```python
from build123d import *

# Parameters (mm, degrees)
SKETCH_1_R                   = 13.5
EXTRUDE_1_DEPTH              = 6
EXTRUDE_START                = -3.8
SKETCH_2_R                   = 19
SKETCH_2_R_2                 = 13.5
EXTRUDE_2_DEPTH              = 3.8
HOLE_WIZARD_M3_1_D           = 3.2
HOLE_WIZARD_M3_1_DEPTH       = 7
HOLE_WIZARD_M3_1_CSINK_D     = 6.5
HOLE_WIZARD_M3_1_CSINK_ANGLE = 90
HOLE_WIZARD_M3_1_TIP         = 0.96137699
F_2_0MM_1_D                  = 2
F_2_0MM_1_DEPTH              = 3.3
F_2_0MM_1_TIP                = 0.600860619
HOLE_WIZARD_M3_1_2_OUTLINE_R = 1.25
HOLE_WIZARD_M3_1_2_DEPTH     = 6
CUT_EXTRUDE_1_DEPTH          = 2
SKETCH_12_R                  = 17.5
SKETCH_12_R_2                = 14.5
CUT_EXTRUDE_3_DEPTH          = 2
EXTRUDE_START_2              = 2
EXTRUDE_3_DEPTH              = 2
CHAMFER_1_SIZE               = 0.5
FILLET_2_R                   = 1
CHAMFER_2_SIZE               = 0.5
CHAMFER_2_SIZE2              = 0.866025404
CHAMFER_3_SIZE               = 0.5


# Read off the part's stored shape, not the designer's step: M3 螺纹孔1
with BuildPart() as part:
    # 草图1 → 凸台-拉伸1 (new body)
    with BuildSketch(Plane.XY):
        Circle(SKETCH_1_R)
    extrude(amount=EXTRUDE_1_DEPTH)

    # 草图2 → 凸台-拉伸2 (add)
    with BuildSketch(Plane.XY.offset(6).offset(EXTRUDE_START)):
        Circle(SKETCH_2_R)
        Circle(SKETCH_2_R_2, mode=Mode.SUBTRACT)
    extrude(amount=EXTRUDE_2_DEPTH)

    # Hole Wizard M3 _1
    with Locations(Plane.XY.offset(6)):
        with Locations((8.660254038, -5), (0, 10), (-8.660254038, -5)):
            CounterSinkHole(HOLE_WIZARD_M3_1_D / 2, HOLE_WIZARD_M3_1_CSINK_D / 2, depth=HOLE_WIZARD_M3_1_DEPTH, counter_sink_angle=HOLE_WIZARD_M3_1_CSINK_ANGLE)
            with Locations((0, 0, -(HOLE_WIZARD_M3_1_DEPTH + HOLE_WIZARD_M3_1_TIP / 2))):  # 118° drill point
                Cone(0, HOLE_WIZARD_M3_1_D / 2, HOLE_WIZARD_M3_1_TIP, mode=Mode.SUBTRACT)

    # Ø2.0mm 暗销孔1
    with Locations(Plane(origin=(0, 0, 0), x_dir=(-1, 0, 0), z_dir=(0, 0, -1))):
        with Locations((8.660254038, 5), (0, -10), (-8.660254038, 5)):
            Hole(F_2_0MM_1_D / 2, depth=F_2_0MM_1_DEPTH)
            with Locations((0, 0, -(F_2_0MM_1_DEPTH + F_2_0MM_1_TIP / 2))):  # 118° drill point
                Cone(0, F_2_0MM_1_D / 2, F_2_0MM_1_TIP, mode=Mode.SUBTRACT)

    # Hole Wizard M3 _1 2 outline → Hole Wizard M3 _1 2 (cut)
    with BuildSketch(Plane.XY):
        with Locations((5.25, 0)):
            Circle(HOLE_WIZARD_M3_1_2_OUTLINE_R)
        with Locations((0, -5.25)):
            Circle(HOLE_WIZARD_M3_1_2_OUTLINE_R)
        with Locations((-5.25, 0)):
            Circle(HOLE_WIZARD_M3_1_2_OUTLINE_R)
        with Locations((0, 5.25)):
            Circle(HOLE_WIZARD_M3_1_2_OUTLINE_R)
    extrude(amount=HOLE_WIZARD_M3_1_2_DEPTH, mode=Mode.SUBTRACT)

    # 草图10 → 切除-拉伸1 (cut)
    with BuildSketch(Plane.XY.offset(6)):
        with BuildLine():
            Line((-2, -1), (-2, 1))
            ThreePointArc((-2, 1), (0, 3), (2, 1))
            Line((2, 1), (2, -1))
            ThreePointArc((2, -1), (0, -3), (-2, -1))
        make_face()
    extrude(amount=-CUT_EXTRUDE_1_DEPTH, mode=Mode.SUBTRACT)

    # 草图12 → 切除-拉伸3 (cut)
    with BuildSketch(Plane(origin=(0, 0, 2.2), x_dir=(-1, 0, 0), z_dir=(0, 0, -1))):
        Circle(SKETCH_12_R)
        Circle(SKETCH_12_R_2, mode=Mode.SUBTRACT)
    extrude(amount=-CUT_EXTRUDE_3_DEPTH, mode=Mode.SUBTRACT)

    # 草图13 → 凸台-拉伸3 (add)
    with BuildSketch(Plane(origin=(0, 0, 4.2), x_dir=(-1, 0, 0), z_dir=(0, 0, -1)).offset(EXTRUDE_START_2)):
        with BuildLine():
            Line((-2.517898576, 14.279712419), (-3.038843109, 17.234135678))
            ThreePointArc((-3.038843109, 17.234135678), (0, 17.5), (3.038843109, 17.234135678))
            Line((3.038843109, 17.234135678), (2.517898576, 14.279712419))
            ThreePointArc((2.517898576, 14.279712419), (0, 14.5), (-2.517898576, 14.279712419))
        make_face()
    extrude(amount=-EXTRUDE_3_DEPTH)

    # 倒角1
    chamfer_1_edges = [part.edges().sort_by_distance(p)[0] for p in [
        (-9.660254038, 5, 0),
        (-1, -10, 0),
        (7.660254038, 5, 0),
    ]]
    chamfer(chamfer_1_edges, length=CHAMFER_1_SIZE)

    # 圆角2
    fillet_2_edges = [part.edges().sort_by_distance(p)[0] for p in [
        (3.038843109, 17.234135678, 3.2),
        (-3.038843109, 17.234135678, 3.2),
        (-2.517898576, 14.279712419, 3.2),
        (2.517898576, 14.279712419, 3.2),
    ]]
    fillet(fillet_2_edges, radius=FILLET_2_R)

    # 倒角2
    chamfer_2_edges = [part.edges().sort_by_distance(p)[0] for p in [
        (0, -3, 6),
        (2, 0, 6),
        (0, 3, 6),
        (-2, 0, 6),
    ]]
    chamfer_2_side = [part.faces().sort_by_distance(p)[0] for p in [
        (-18.462598846, 0, 6),
    ]]
    chamfer(chamfer_2_edges, length=CHAMFER_2_SIZE, length2=CHAMFER_2_SIZE2, reference=chamfer_2_side[0])

    # 倒角3
    chamfer_3_edges = [part.edges().sort_by_distance(p)[0] for p in [
        (-2.772933692, 15.726088432, 2.2),
        (0, -14.5, 2.2),
        (0, -17.5, 2.2),
        (2.772933692, 15.726088432, 2.2),
        (-2.833509711, 14.512231288, 2.2),
        (-3.296257199, 16.88197424, 2.2),
        (3.296257199, 16.88197424, 2.2),
        (2.833509711, 14.512231288, 2.2),
        (-13.5, 0, 0),
        (-19, 0, 2.2),
        (-19, 0, 6),
    ]]
    chamfer(chamfer_3_edges, length=CHAMFER_3_SIZE)


solid = part.part
```
For this review, take the finished solid that the model builds, in its own axes (mm). A direction names the side the tool comes from. Give positions to 0.01 mm unless a question says otherwise; leave off trailing zeros. Answer as a JSON object with one key per item and string values. Group by question number.
Item 1: Consider section A-A on z = 1.45. Count the separate pieces of the cut face and the enclosed holes in it, plus the area to 3 significant figures.
Item 2: For probe 1 along Y at (x, z) = (0, 3.25); probe 2 along Y at (x, z) = (0, 1.2); probe 3 along X at (y, z) = (5, 2.7), list the stretches that pass through material, from the lowest coordinate up. Write a range as [from, to].
Item 3: For pin 1 Ø1.8 at (x, y) = (-8.66, 5) entering from -Z; pin 2 Ø2.5 at (x, y) = (8.66, 5) entering from -Z; pin 3 Ø1 at (y, z) = (12, 4) entering from +X, all flat-tipped, find the tip position at first contact; note any pin that passes through.
Item 4: Tool access review of faces 1 (the flat face through (-2.774, 15.733, 3.44)), 2 (the cylindrical face through (0.35, 8.44, 2.14)), 3 (the cylindrical face through (0, -3, 4.6)): name each direction out of +Z, -Z, +X, -X, +Y, -Y from which nothing blocks a thin tool from reaching the whole face with its end or side.
Check result:
{
 "1": {"separate pieces": "1", "enclosed holes": "10", "area": "519 mm^2"},
 "2": {"probe 1": "y = [-19, -17.5], [-14.5, -11], [-9, -6.5], [-4, 4], [6.5, 8.4], [11.6, 19]", "probe 2": "y = [-13.5, -11], [-9, -6.5], [-4, 4], [6.5, 8.4], [11.6, 13.5]", "probe 3": "x = [-18.33, -16.77], [-13.61, -9.66], [-7.66, -1.22], [1.22, 7.66], [9.66, 13.61], [16.77, 18.33]"},
 "3": {"pin 1": "stops at z = 3.36", "pin 2": "stops at z = 0.25", "pin 3": "stops at x = 15.12"},
 "4": {"face 1": "-Z", "face 2": "+Z, -Z", "face 3": "+Z"}
}
